from build123d import *

# Parameters (mm, degrees)
BOSS_EXTRUDE2_DEPTH = 10
BOSS_EXTRUDE3_DEPTH = 5
FILLET1_R           = 10
SKETCH3_W           = 150
SKETCH3_H           = 15
BOSS_EXTRUDE4_DEPTH = 17.5
SKETCH5_W           = 51
SKETCH5_H           = 14.230744396
CUT_EXTRUDE1_DEPTH  = 3
FILLET2_R           = 5


with BuildPart() as part:
    # Sketch1 → Boss-Extrude2 (new body)
    with BuildSketch(Plane.XY):
        with BuildLine():
            Line((40, 52.5), (40, 80))
            Line((40, 80), (45, 80))
            Line((45, 80), (45, 52.5))
            ThreePointArc((45, 52.5), (40.606601718, 41.893398282), (30, 37.5))
            Line((30, 37.5), (-70, 37.5))
            ThreePointArc((-70, 37.5), (-80.606601718, 41.893398282), (-85, 52.5))
            Line((-85, 52.5), (-85, 80))
            Line((-85, 80), (-80, 80))
            Line((-80, 80), (-80, 52.5))
            ThreePointArc((-80, 52.5), (-77.071067812, 45.428932188), (-70, 42.5))
            Line((-70, 42.5), (30, 42.5))
            ThreePointArc((30, 42.5), (37.071067812, 45.428932188), (40, 52.5))
        make_face()
    extrude(amount=BOSS_EXTRUDE2_DEPTH)

    # Sketch2 → Boss-Extrude3 (add)
    with BuildSketch(Plane.XY.offset(10)):
        with BuildLine():
            Line((45, 52.5), (45, 80))
            Line((45, 80), (-85, 80))
            Line((-85, 80), (-85, 52.5))
            ThreePointArc((-85, 52.5), (-80.606601718, 41.893398282), (-70, 37.5))
            Line((-70, 37.5), (30, 37.5))
            ThreePointArc((30, 37.5), (40.606601718, 41.893398282), (45, 52.5))
        make_face()
    extrude(amount=BOSS_EXTRUDE3_DEPTH)

    # Fillet1
    fillet1_edges = [part.edges().sort_by_distance(p)[0] for p in [
        (-80, 66.25, 10),
        (-77.071067812, 45.428932188, 10),
        (-20, 42.5, 10),
        (37.071067812, 45.428932188, 10),
        (40, 66.25, 10),
    ]]
    fillet(fillet1_edges, radius=FILLET1_R - 0.0001)  # a hair under: the kernel refuses the full size

    # Sketch3 → Boss-Extrude4 (add)
    with BuildSketch(Plane(origin=(0, 80, 0), x_dir=(1, 0, 0), z_dir=(0, 1, 0))):
        with Locations((-20, -7.5)):
            Rectangle(SKETCH3_W, SKETCH3_H)
    extrude(amount=BOSS_EXTRUDE4_DEPTH)

    # Sketch5 → Cut-Extrude1 (cut)
    with BuildSketch(Plane(origin=(0, 0, 0), x_dir=(-1, 0, 0), z_dir=(0, 0, -1))):
        with Locations((-25.5, 87.115372198)):
            Rectangle(SKETCH5_W, SKETCH5_H)
        with Locations((65.5, 87.115372198)):
            Rectangle(SKETCH5_W, SKETCH5_H)
    extrude(amount=-CUT_EXTRUDE1_DEPTH, mode=Mode.SUBTRACT)

    # Fillet2
    fillet2_edges = [part.edges().sort_by_distance(p)[0] for p in [
        (-20, 37.5, 15),
        (-80.606601718, 41.893398282, 15),
        (-85, 66.25, 15),
        (-90, 80, 15),
        (-95, 88.75, 15),
        (-20, 97.5, 15),
        (55, 88.75, 15),
        (50, 80, 15),
        (45, 66.25, 15),
        (40.606601718, 41.893398282, 15),
        (-95, 97.5, 7.5),
        (55, 97.5, 7.5),
    ]]
    fillet(fillet2_edges, radius=FILLET2_R)


solid = part.part
Verification items for the finished model (mm, model axes). A direction names the side the tool comes from. Give positions to 0.01 mm unless a question says otherwise; leave off trailing zeros. Write each loop counter-clockwise with the first axis right and the second up, starting at its lowest first coordinate (ties: lowest second). Pieces come first, ordered by that corner, then holes. Notation, with made-up numbers: (58, 82.5) -> (102, 82.5) arc R16 ccw to (102, 111.5) -> close; hole circle Ø5 at (-12, -8). An arc over 180 degrees is marked (long way). Use CSV: the item, a comma, the result in double quotes.
(1) Material ranges on L1, parallel to Y at x = 6, z = 10.5; L2, parallel to Z at x = 1, y = 75; L3, parallel to Y at x = -66.5, z = 8.75, recorded low to high.
Derived:
L1,"y = 37.53 to 97.47"
L2,"z = 10 to 15"
L3,"y = 37.5 to 47.66, 80 to 97.5"
(2) Set-up check for faces 4 (the flat face through (-40, 87, 1)), 5 (the flat face through (-85, 66, 5)), 6 (the cylindrical face through (48, 82, 14)): record each of +Z, -Z, +X, -X, +Y, -Y from which the full face is reachable in a straight line by a thin tool's end or side.
Derived:
face 4,"-Z"
face 5,"+Z, -Z, -X, -Y"
face 6,"+Z, +X, -Y"
(3) Go/stop test with flat-tipped pins: pin 1 (8.5 mm diameter, centred on x = -10.5, y = 73, fed in from -Z); pin 2 (11.5 mm diameter, centred on x = -68, y = 84, fed in from -Z); pin 3 (3 mm diameter, centred on y = 68, z = 3.5, fed in from -X). Record where each tip stops, or that it passes through.
Derived:
pin 1,"stops at z = 10"
pin 2,"stops at z = 3"
pin 3,"stops at x = -85"
(4) Sectioned sample at C-C (z = 12). Record the cut outline in (x, y).
Derived:
outline,"(-94.58, 80.42) -> (-84.58, 80.42) -> (-84.58, 52.5) arc R14.58 ccw to (-70, 37.92) -> (30, 37.92) arc R14.58 ccw to (44.58, 52.5) -> (44.58, 80.42) -> (54.58, 80.42) -> (54.58, 92.5) arc R4.58 ccw to (50, 97.08) -> (-90, 97.08) arc R4.58 ccw to (-94.58, 92.5) -> close"
(5) Release check for a two-part mould opening along X. For faces 1 (the flat face through (26, 94.231, 1)), 2 (the cylindrical face through (-94, 88, 13)), 3 (the flat face through (55, 86, 5)) record: +X half, -X half, draft (parallel to the pull), parting line (faces both ways), or undercut.
Derived:
face 1,"undercut"
face 2,"-X half"
face 3,"+X half"
